For this review, take the finished solid that the model builds, in its own axes (mm). A direction names the side the tool comes from. Give positions to 0.01 mm unless a question says otherwise; leave off trailing zeros. Loops run counter-clockwise (first coordinate to the right, second up) from the corner with the lowest first, then second, coordinate; pieces in that order, holes last. Notation, with made-up numbers: (37, 7.5) - (49, 7.5) arc R6 cw to (49, 18.5) - close; hole circle Ø3 at (22, -12). An arc over 180 degrees is marked (long way). Answer in a Markdown table with one row per item.
```python
from build123d import *

# Parameters (mm, degrees)
SKETCH1_R                            = 2.0193
BOSS_EXTRUDE1_DEPTH                  = 14.3256
F_10_32_TAPPED_HOLE1_D               = 4.0386
F_10_32_TAPPED_HOLE1_DEPTH           = 11.938
F_10_32_TAPPED_HOLE1_TIP             = 1.213317848
F_10_32_TAPPED_HOLE1_ON_FACE_2_D     = 4.0386
F_10_32_TAPPED_HOLE1_ON_FACE_2_DEPTH = 11.938
F_10_32_TAPPED_HOLE1_ON_FACE_2_TIP   = 1.213317848
SKETCH4_R                            = 8.89
SKETCH4_R_2                          = 6.35
CUT_EXTRUDE_THIN1_DEPTH              = 7.9375


with BuildPart() as part:
    # Sketch1 → Boss-Extrude1 (new, symmetric)
    with BuildSketch(Plane.XY):
        Polygon((7.332348419, 0), (3.666174209, 6.35), (-3.666174209, 6.35), (-7.332348419, 0), (-3.666174209, -6.35), (3.666174209, -6.35), align=None)
        Circle(SKETCH1_R, mode=Mode.SUBTRACT)
    extrude(amount=BOSS_EXTRUDE1_DEPTH, both=True)

    # #10-32 Tapped Hole1
    with Locations(Plane.XY.offset(14.3256)):
        with Locations((0, 0)):
            Hole(F_10_32_TAPPED_HOLE1_D / 2, depth=F_10_32_TAPPED_HOLE1_DEPTH)
            with Locations((0, 0, -(F_10_32_TAPPED_HOLE1_DEPTH + F_10_32_TAPPED_HOLE1_TIP / 2))):  # 118° drill point
                Cone(0, F_10_32_TAPPED_HOLE1_D / 2, F_10_32_TAPPED_HOLE1_TIP, mode=Mode.SUBTRACT)

    # #10-32 Tapped Hole1 on face 2
    with Locations(Plane.XY.offset(-14.3256)):
        with Locations((0, 0)):
            Hole(F_10_32_TAPPED_HOLE1_ON_FACE_2_D / 2, depth=F_10_32_TAPPED_HOLE1_ON_FACE_2_DEPTH)
            with Locations((0, 0, -(F_10_32_TAPPED_HOLE1_ON_FACE_2_DEPTH + F_10_32_TAPPED_HOLE1_ON_FACE_2_TIP / 2))):  # 118° drill point
                Cone(0, F_10_32_TAPPED_HOLE1_ON_FACE_2_D / 2, F_10_32_TAPPED_HOLE1_ON_FACE_2_TIP, mode=Mode.SUBTRACT)

    # Sketch4 → Cut-Extrude-Thin1 (cut)
    with BuildSketch(Plane.XY.offset(14.3256)):
        Circle(SKETCH4_R)
        Circle(SKETCH4_R_2, mode=Mode.SUBTRACT)
    cut_extrude_thin1 = extrude(amount=-CUT_EXTRUDE_THIN1_DEPTH, mode=Mode.SUBTRACT)

    # Mirror1: Cut-Extrude-Thin1 across plane
    add(cut_extrude_thin1.mirror(Plane.XY), mode=Mode.SUBTRACT)


solid = part.part
```
1. Wall thickness on line 1 (Y direction, x = 0, z = -8.5); line 2 (Y direction, x = 1.75, z = -12.25): over which ranges is each line inside the solid? List them lowest first. Write a range as [from, to].
Values:
| item | result |
|---|---|
| line 1 | y = [-6.35, -2.02], [2.02, 6.35] |
| line 2 | y = [-6.1, -1.01], [1.01, 6.1] |
2. We need section D-D, the plane y = 5.25. Give the boundary of the cut face in (x, z).
Values:
| item | result |
|---|---|
| outline | (-4.3, -6.39) - (-3.57, -6.39) - (-3.57, -14.33) - (3.57, -14.33) - (3.57, -6.39) - (4.3, -6.39) - (4.3, 6.39) - (3.57, 6.39) - (3.57, 14.33) - (-3.57, 14.33) - (-3.57, 6.39) - (-4.3, 6.39) - close |
3. Mouldability with a two-part tool opening along Y and no side actions: class faces 4 (the face through (-7, 0, -6.388)), 5 (the face through (0, 6.35, 0)), 6 (the face through (1.926, 0.607, -0.201)) as released by +Y, released by -Y, zero draft, split by the parting line, or undercut.
Values:
| item | result |
|---|---|
| face 4 | zero draft |
| face 5 | released by +Y |
| face 6 | undercut |
4. For faces 1 (the face through (3, -6, -6.388)), 2 (the face through (3, 6, -6.388)), 3 (the face through (-1.38, -6.2, 10.41)), list the 3-axis set-ups (+Z, -Z, +X, -X, +Y, -Y) from which the entire face can be reached by the end or side of a thin tool; tool diameter is ignored.
Values:
| item | result |
|---|---|
| face 1 | -Z, +X, -Y |
| face 2 | -Z, +X, +Y |
| face 3 | +Z |
5. We need section C-C, the plane x = 3. Give the boundary of the cut face in (y, z).
Values:
| item | result |
|---|---|
| outline | (-6.35, -6.39) - (-5.6, -6.39) - (-5.6, -14.33) - (5.6, -14.33) - (5.6, -6.39) - (6.35, -6.39) - (6.35, 6.39) - (5.6, 6.39) - (5.6, 14.33) - (-5.6, 14.33) - (-5.6, 6.39) - (-6.35, 6.39) - close |
6. We need section A-A, the plane z = -5.75. Give the boundary of the cut face in (x, y), and give its area (3 significant figures).
Values:
| item | result |
|---|---|
| outline | (-7.33, 0) - (-3.67, -6.35) - (3.67, -6.35) - (7.33, 0) - (3.67, 6.35) - (-3.67, 6.35) - close; hole circle Ø4.04 at (0, 0) |
| area | 127 mm^2 |
7. Clearance check with flat-ended pins moving along their axes: pin 1 (2.5 mm diameter, centred on x = 0, y = 0, fed in from +Z); pin 2 (3 mm diameter, centred on x = 2, z = 8, fed in from -Y); pin 3 (0.5 mm diameter, centred on x = 6.5, y = 1.5, fed in from -Z); pin 4 (5 mm diameter, centred on y = 2.5, z = 11, fed in from -X). State where each tip first meets the part, or that it passes through.
Values:
| item | result |
|---|---|
| pin 1 | passes through |
| pin 2 | stops at y = -6.33 |
| pin 3 | stops at z = -6.39 |
| pin 4 | stops at x = -6.35 |
8. We need section B-B, the plane y = 0.75. Give the boundary of the cut face in (x, z).
Values:
| item | result |
|---|---|
| outline | (-6.9, -6.39) - (-6.31, -6.39) - (-6.31, -14.33) - (-1.87, -14.33) - (-1.87, 14.33) - (-6.31, 14.33) - (-6.31, 6.39) - (-6.9, 6.39) - close; (1.87, -14.33) - (6.31, -14.33) - (6.31, -6.39) - (6.9, -6.39) - (6.9, 6.39) - (6.31, 6.39) - (6.31, 14.33) - (1.87, 14.33) - close |
